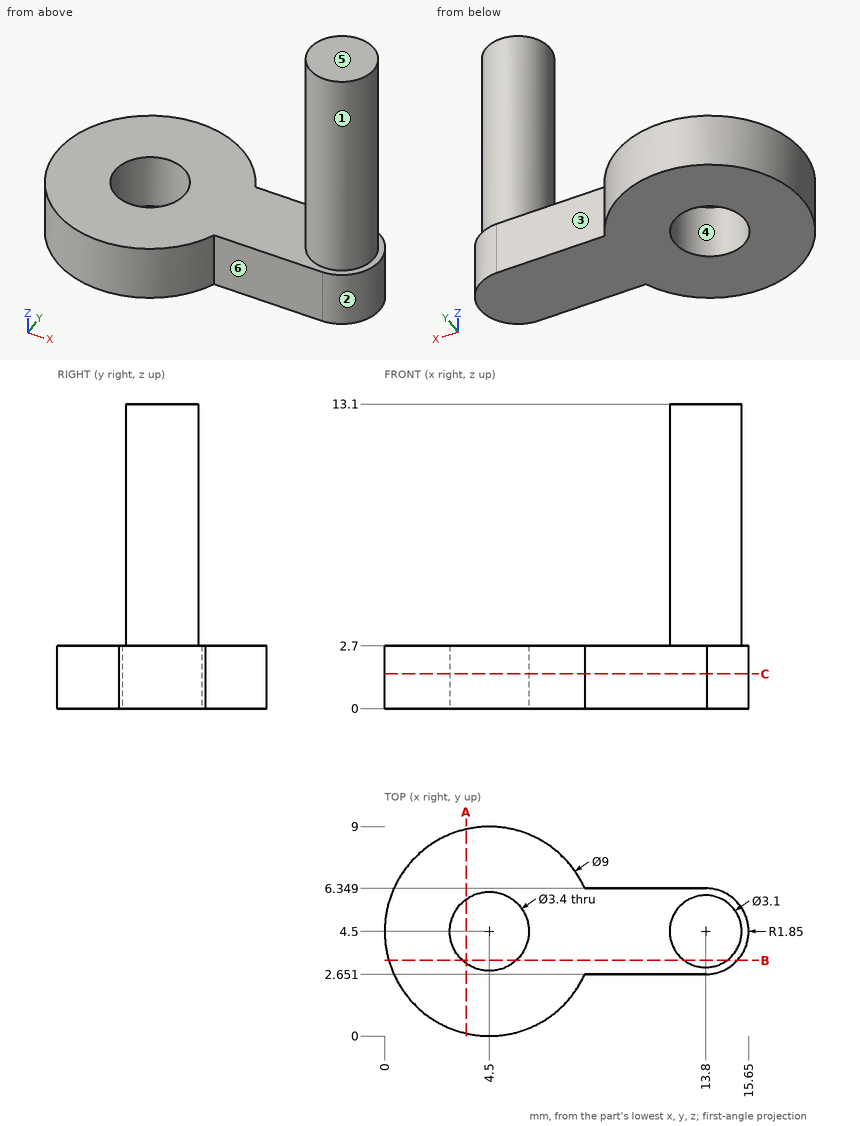
Can you work these out from the drawing? Everything is in mm from the part's minimum corner. A direction names the side the tool comes from. Give positions to 0.01 mm unless a question says otherwise; leave off trailing zeros. Order: outer loops, then holes, each group sorted by start corner. A loop starts at its lowest first (then second) coordinate and runs counter-clockwise, first axis right, second up. Notation, with made-up numbers: M 26.25,39 L 62.25,39 A13 ccw 62.25,45 Z; hole C 4,28 d5. An arc over 180 degrees is marked long. One line per question, with ' | ' between items.
1. We'd pull the mould along Y, two halves only. Please class the marked faces 4, 5 and 6: +Y half, -Y half, draft (parallel to the pull), parting line (faces both ways), or undercut.
Results:
face 4: undercut | face 5: draft | face 6: -Y half
2. For the marked faces 1, 2 and 3, which set-ups out of +Z, -Z, +X, -X, +Y, -Y let a thin tool reach every point of the face, with its end or its side?
Results:
face 1: +Z | face 2: +Z, -Z, +X | face 3: +Z, -Z, +X, +Y
3. I'm going to push flat-ended pins straight in: pin 1 (3 mm diameter, centred on y = 7.5, z = 2, fed in from -X); pin 2 (2 mm diameter, centred on x = 10, z = 3, fed in from -Y); pin 3 (2 mm diameter, centred on x = 11, z = 0.5, fed in from +Y). Where does each tip first touch, or does it pass through?
Results:
pin 1: x = 0.26 | pin 2: y = 2.65 | pin 3: y = 6.35
4. I want a section at C-C (z = 1.5). List the corners of the cut face in (x, y) for me.
Results:
outline: M 8.6,2.65 L 13.85,2.65 A1.85 ccw 13.85,6.35 L 8.6,6.35 A4.5 ccw long Z; hole C 4.5,4.5 d3.4
5. I want a section at A-A (x = 3.5). List the corners of the cut face in (y, z) for me (1 decimal), and give its area (3 significant figures).
Results:
outline: M 0.1,0 L 3.1,0 L 3.1,2.7 L 0.1,2.7 Z; M 5.9,0 L 8.9,0 L 8.9,2.7 L 5.9,2.7 Z | area: 16.3 mm²
6. If I drill on line 1 (X direction, y = 4.5, z = 1); line 2 (Z direction, x = 12, y = 6); line 3 (X direction, y = 6.5, z = 1.5), over which ranges is the centre line in solid material (lowest first)?
Results:
line 1: 0 to 2.8, 6.2 to 15.65 | line 2: 0 to 2.7 | line 3: 0.47 to 8.53
7. I want a section at B-B (y = 3.25). List the corners of the cut face in (x, z) for me.
Results:
outline: M 0.18,0 L 3.35,0 L 3.35,2.7 L 0.18,2.7 Z; M 5.65,0 L 15.16,0 L 15.16,2.7 L 14.72,2.7 L 14.72,13.1 L 12.88,13.1 L 12.88,2.7 L 5.65,2.7 Z
